```python
from build123d import *

# Parameters (mm, degrees)
SKETCH1_W           = 40
SKETCH1_H           = 29
BOSS_EXTRUDE1_DEPTH = 20
FILLET2_R           = 6.5
SKETCH3_W           = 48.982601016
SKETCH3_H           = 39.309165856
CUT_EXTRUDE1_DEPTH  = 14.5
SHELL1_T            = -2
BOSS_EXTRUDE3_DEPTH = 3
FILLET3_R           = 0.2
SKETCH6_R           = 4.5
CUT_EXTRUDE2_DEPTH  = 10.5000001
CHAMFER1_SIZE       = 0.5


with BuildPart() as part:
    # Sketch1 → Boss-Extrude1 (new body)
    with BuildSketch(Plane(origin=(0, 0, 0), x_dir=(1, 0, 0), z_dir=(0, 1, 0))):
        Rectangle(SKETCH1_W, SKETCH1_H)
    extrude(amount=BOSS_EXTRUDE1_DEPTH)

    # Fillet2
    fillet2_edges = [part.edges().sort_by_distance(p)[0] for p in [
        (-20, 20, 0),
        (0, 20, 14.5),
        (20, 20, 0),
        (0, 0, 14.5),
        (-20, 0, 0),
        (0, 0, -14.5),
        (20, 0, 0),
        (20, 10, 14.5),
        (-20, 10, 14.5),
        (-20, 10, -14.5),
        (20, 10, -14.5),
        (0, 20, -14.5),
    ]]
    fillet(fillet2_edges, radius=FILLET2_R)

    # Sketch3 → Cut-Extrude1 (cut, through all)
    with BuildSketch(Plane(origin=(0, 13.5, 0), x_dir=(1, 0, 0), z_dir=(0, 1, 0))):
        Rectangle(SKETCH3_W, SKETCH3_H)
    extrude(amount=-CUT_EXTRUDE1_DEPTH, mode=Mode.SUBTRACT)

    # Shell1
    shell1_openings = [part.faces().sort_by_distance(p)[0] for p in [
        (0, 13.5, 0),
    ]]
    offset(amount=SHELL1_T, openings=shell1_openings)

    # Sketch5 → Boss-Extrude3 (add)
    with BuildSketch(Plane.XZ.offset(-13.5)):
        with BuildLine():
            Line((-14.3, 13.845511098), (-14.3, 13.340411969))
            ThreePointArc((-14.3, 13.340411969), (-17.318376618, 11.818376618), (-18.840411969, 8.8))
            Line((-18.840411969, 8.8), (-19.345511098, 8.8))
            ThreePointArc((-19.345511098, 8.8), (-17.671930009, 12.171930009), (-14.3, 13.845511098))
        make_face()
        with BuildLine():
            Line((-14.3, -13.845511098), (-14.3, -13.340411969))
            ThreePointArc((-14.3, -13.340411969), (-17.318376618, -11.818376618), (-18.840411969, -8.8))
            Line((-18.840411969, -8.8), (-19.345511098, -8.8))
            ThreePointArc((-19.345511098, -8.8), (-17.671930009, -12.171930009), (-14.3, -13.845511098))
        make_face()
        with BuildLine():
            Line((14.3, -13.845511098), (14.3, -13.340411969))
            ThreePointArc((14.3, -13.340411969), (17.318376618, -11.818376618), (18.840411969, -8.8))
            Line((18.840411969, -8.8), (19.345511098, -8.8))
            ThreePointArc((19.345511098, -8.8), (17.671930009, -12.171930009), (14.3, -13.845511098))
        make_face()
        with BuildLine():
            Line((19.345511098, 8.8), (18.840411969, 8.8))
            ThreePointArc((18.840411969, 8.8), (17.318376618, 11.818376618), (14.3, 13.340411969))
            Line((14.3, 13.340411969), (14.3, 13.845511098))
            ThreePointArc((14.3, 13.845511098), (17.671930009, 12.171930009), (19.345511098, 8.8))
        make_face()
    extrude(amount=BOSS_EXTRUDE3_DEPTH)

    # Fillet3
    fillet3_edges = [part.edges().sort_by_distance(p)[0] for p in [
        (-17.318376618, 10.5, 11.818376618),
        (-17.671930009, 10.5, 12.171930009),
        (-17.318376618, 10.5, -11.818376618),
        (-17.671930009, 10.5, -12.171930009),
        (17.318376618, 10.5, 11.818376618),
        (17.671930009, 10.5, 12.171930009),
        (17.671930009, 10.5, -12.171930009),
        (-14.3, 10.5, 13.592961534),
        (-19.092961534, 10.5, 8.8),
        (-19.092961534, 10.5, -8.8),
        (-14.3, 10.5, -13.592961534),
        (19.092961534, 10.5, 8.8),
        (14.3, 10.5, 13.592961534),
    ]]
    fillet(fillet3_edges, radius=FILLET3_R)

    # Sketch6 → Cut-Extrude2 (cut, through all)
    with BuildSketch(Plane(origin=(0, 20, 0), x_dir=(1, 0, 0), z_dir=(0, 1, 0))):
        with Locations(Location((-8.25, 0, 0), (0, 0, 270))):  # turned: the seam where the file's is
            Circle(SKETCH6_R)
        with Locations(Location((8.25, 0, 0), (0, 0, 270))):  # turned: the seam where the file's is
            Circle(SKETCH6_R)
    extrude(amount=-CUT_EXTRUDE2_DEPTH, mode=Mode.SUBTRACT)

    # Chamfer1
    chamfer1_edges = [part.edges().sort_by_distance(p)[0] for p in [
        (-8.25, 20, -4.5),
        (8.25, 20, -4.5),
    ]]
    chamfer(chamfer1_edges, length=CHAMFER1_SIZE)


solid = part.part
```
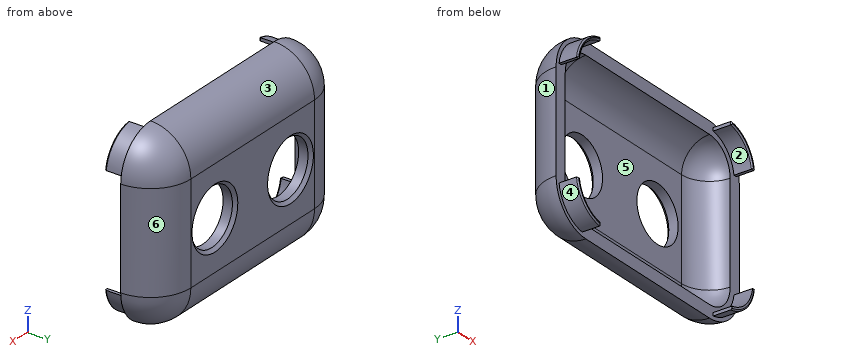
The listing builds one solid part. Answer for the finished solid, in the listing's coordinates (mm). Face numbers are marked on the shaded views. A direction names the side the tool comes from. Coordinates: 2 decimals unless noted, no trailing zeros. Write each loop counter-clockwise with the first axis right and the second up, starting at its lowest first coordinate (ties: lowest second). Pieces come first, ordered by that corner, then holes. Notation, with made-up numbers: M -17.75,78.5 L 22.25,78.5 A18 cw 22.25,113.5 Z; hole C 64.5,25 d9. An arc over 180 degrees is marked long. Use a Markdown table: item, result. Add a question column.
1. Which of the six approach directions +Z, -Z, +X, -X, +Y, -Y give full straight-line access (tool end or side, diameter ignored) to the marked faces 4, 5 and 6?
2. Section B-B (x = 8.25) is taken. Give the vertices of the cut face in (y, z), plus the area to 3 significant figures.
3. Section A-A (z = 0) is taken. Give the vertices of the cut face in (x, y), plus the area to 3 significant figures.
4. For a pull along X with two mould halves and no side action, classify the marked faces 1, 2 and 3 as +X half, -X half, draft (parallel to the pull), parting line (faces both ways), or undercut.
5. Section C-C (y = 16) is taken. Give the vertices of the cut face in (x, z), plus the area to 3 significant figures.
6. Given P1, Ø0.6, axis at y = 11.5, z = 13.5, coming from the -X side; P2, Ø3, axis at x = 10.5, z = 1, coming from the -Y side; P3, Ø4, axis at y = 17, z = 0, coming from the -X side; P4, Ø14.5, axis at x = -8.25, z = 0, coming from the -Y side, each flat-ended and moving along its own axis, determine where each tip first touches the part or whether it passes through.
7. Straight lines are drawn through the part: line 1 along X through (y, z) = (19.1, 0); line 2 along X through (y, z) = (18.6, 0); line 3 along X through (y, z) = (14, 6.75). For each, find the intervals that lie inside material, in ascending order. Write a range as [from, to].
Data:
| question | item | result |
|---|---|---|
| 1 | face 4 | -Z, -X, -Y |
| 1 | face 5 | -Y |
| 1 | face 6 | +Z, -Z, +X, +Y |
| 2 | outline | M 13.5,-14.5 A6.5 ccw 20,-8 L 20,-5 L 19.5,-4.5 L 18,-4.5 L 18,-8 A4.5 cw 13.5,-12.5 Z; M 13.5,12.5 A4.5 cw 18,8 L 18,4.5 L 19.5,4.5 L 20,5 L 20,8 A6.5 ccw 13.5,14.5 Z |
| 2 | area | 48.3 mm2 |
| 3 | outline | M -20,13.5 L -18,13.5 A4.5 cw -13.5,18 L -12.75,18 L -12.75,19.5 L -13.25,20 L -13.5,20 A6.5 ccw Z; M -3.75,18 L 3.75,18 L 3.75,19.5 L 3.25,20 L -3.25,20 L -3.75,19.5 Z; M 12.75,18 L 13.5,18 A4.5 cw 18,13.5 L 20,13.5 A6.5 ccw 13.5,20 L 13.25,20 L 12.75,19.5 Z |
| 3 | area | 52.1 mm2 |
| 4 | face 1 | -X half |
| 4 | face 2 | undercut |
| 4 | face 3 | draft |
| 5 | outline | M -19.5,-8 A6 ccw -13.5,-14 L 13.5,-14 A6 ccw 19.5,-8 L 19.5,8 A6 ccw 13.5,14 L -13.5,14 A6 ccw -19.5,8 Z; hole M -17.24,-8 A3.74 ccw -13.5,-11.74 L 13.5,-11.74 A3.74 ccw 17.24,-8 L 17.24,8 A3.74 ccw 13.5,11.74 L -13.5,11.74 A3.74 ccw -17.24,8 Z |
| 5 | area | 263 mm2 |
| 6 | P1 | stops at x = -16.29 |
| 6 | P2 | passes through |
| 6 | P3 | stops at x = -19.82 |
| 6 | P4 | stops at y = 17.53 |
| 7 | line 1 | x = [-16.8, -12.75], [-3.75, 3.75], [12.75, 16.8] |
| 7 | line 2 | x = [-17.53, -12.75], [-3.75, 3.75], [12.75, 17.53] |
| 7 | line 3 | x = [-19.98, -17.97], [17.97, 19.98] |
